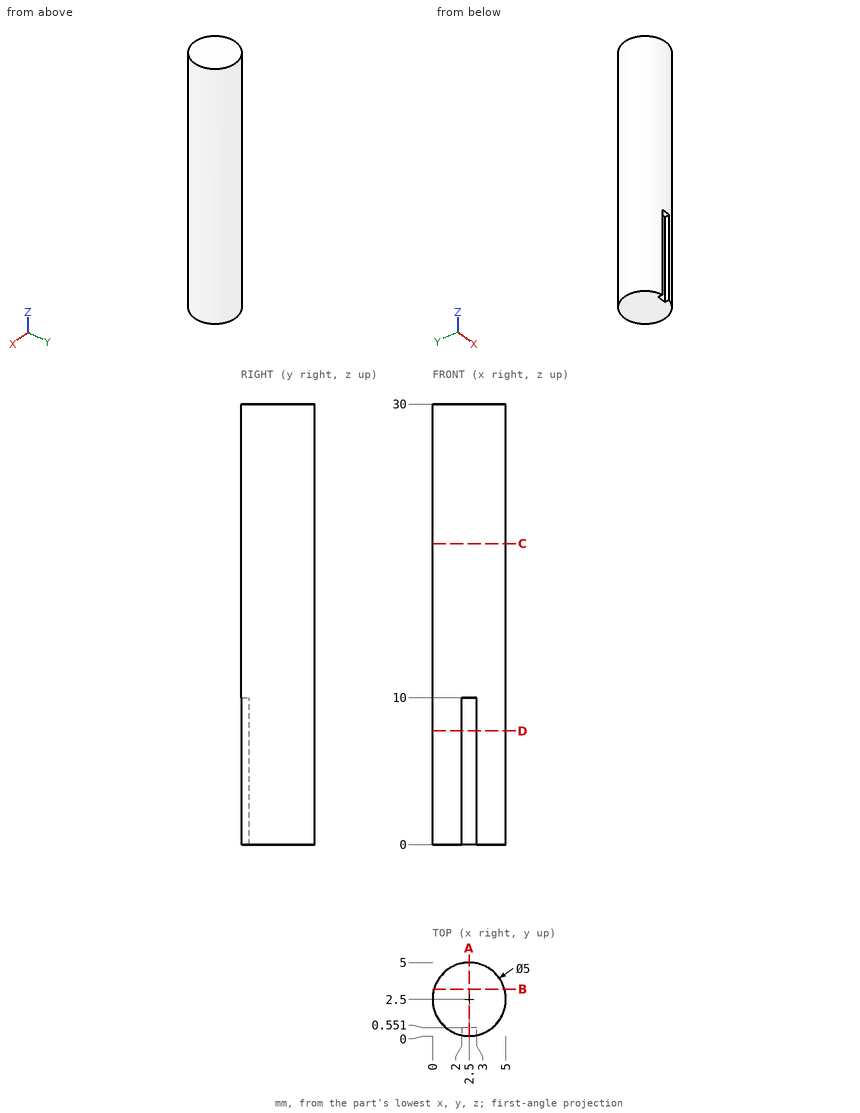
For this review, use the dimensioned drawing (mm, ordinates from the lowest corner) and the shaded views. Round coordinates to 2 decimals unless told otherwise and drop trailing zeros. Write each loop counter-clockwise with the first axis right and the second up, starting at its lowest first coordinate (ties: lowest second). Pieces come first, ordered by that corner, then holes. Notation, with made-up numbers: M 36.5,64.25 L 44.5,64.25 A30 ccw 44.5,92.25 Z; hole C 40,72 d10. An arc over 180 degrees is marked long. Use CSV: the item, a comma, the result in double quotes. Start each with the question number.
(1) We need section C-C, the plane z = 20.5. State the section outline as (x, y) points.
(2) We need section D-D, the plane z = 7.75. State the section outline as (x, y) points, then the cut area to 3 significant figures.
(3) We need section B-B, the plane y = 3.2. State the section outline as (x, z) points, then the cut area to 3 significant figures.
(4) We need section A-A, the plane x = 2.5. State the section outline as (y, z) points.
(5) For line 1 along X through (y, z) = (2.2, 19); line 2 along Y through (x, z) = (3.15, 27.75) (1 decimal); line 3 along Y through (x, z) = (1.25, 26) (1 decimal), list the stretches that pass through material, from the lowest coordinate up.
(6) Clearance check with flat-ended pins moving along their axes: P1, Ø2, axis at x = 1, z = 12.5, coming from the +Y side; P2, Ø0.5, axis at x = 2.5, z = 3, coming from the -Y side; P3, Ø0.6, axis at y = 0, z = 6.5, coming from the -X side (1 decimal). State where each tip first meets the part, or that it passes through.
Findings:
1,outline,"C 2.5,2.5 d5"
2,outline,"M 2,0.05 L 2,0.55 L 3,0.55 L 3,0.05 A2.5 ccw long Z"
2,area,"19.1 mm^2"
3,outline,"M 0.1,0 L 4.9,0 L 4.9,30 L 0.1,30 Z"
3,area,"144 mm^2"
4,outline,"M 0,10 L 0.55,10 L 0.55,0 L 5,0 L 5,30 L 0,30 Z"
5,line 1,"0.02 to 4.98"
5,line 2,"0.1 to 4.9"
5,line 3,"0.3 to 4.7"
6,P1,"y = 4.95"
6,P2,"y = 0.55"
6,P3,"x = 1.3"
